Here's the drawing with two shaded views (mm, measured from the low corner). I have some questions. Coordinates: 2 decimals unless noted, no trailing zeros. Loops run counter-clockwise (first coordinate to the right, second up) from the corner with the lowest first, then second, coordinate; pieces in that order, holes last.
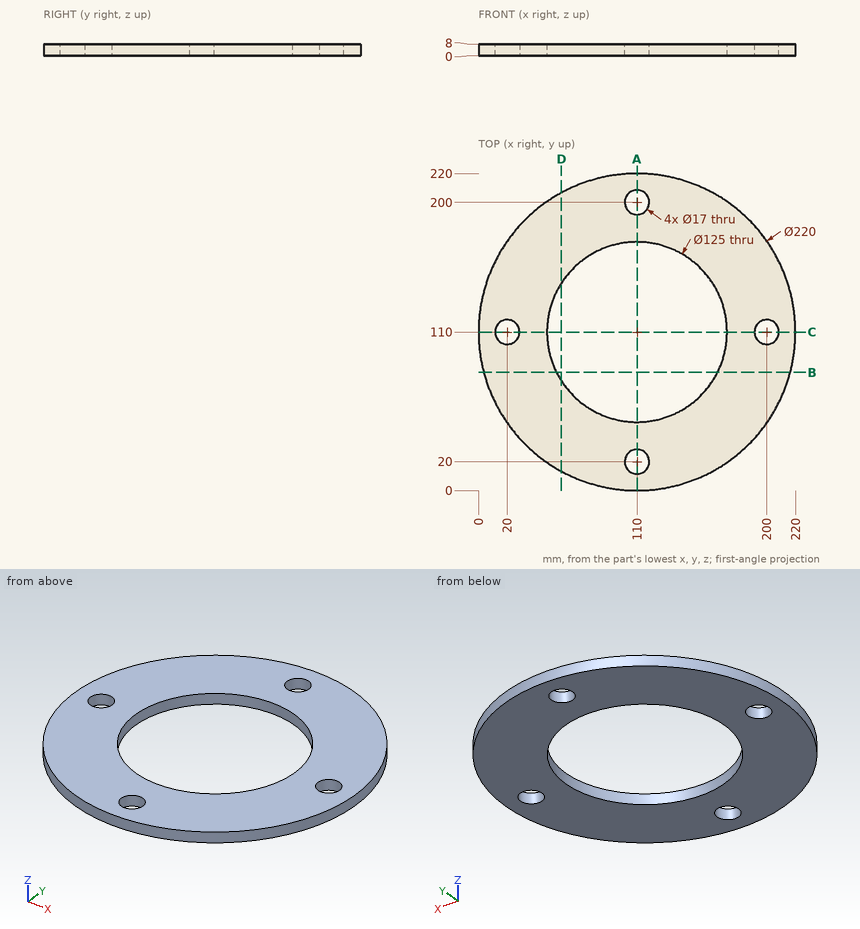
Q1. Will these pins go through, and if not, where does the flat tip stop? P1, Ø3, axis at y = 196.5, z = 6, coming from the -X side; P2, Ø13.5, axis at x = 110, y = 20, coming from the -Z side; P3, Ø1, axis at y = 34.5, z = 3.5, coming from the +X side; P4, Ø1.5, axis at x = 193.5, z = 6, coming from the +Y side.
Q2. Suppose I cut it at B-B on y = 82. Write out the boundary of the cut face in (x, z).
Q3. Suppose I cut it at A-A on x = 110. Write out the boundary of the cut face in (y, z), and give its area (3 significant figures).
Q4. Suppose I cut it at D-D on x = 57.5. Write out the boundary of the cut face in (y, z), and give its area (3 significant figures).
Q5. Please list where these lines run through material, in increasing order: probe 1 along X at (y, z) = (105, 6.75); probe 2 along X at (y, z) = (52, 1); probe 3 along X at (y, z) = (207, 6).
Check values:
1. P1: stops at x = 40.18
1. P2: passes through
1. P3: stops at x = 190.47
1. P4: stops at y = 182.47
2. outline: (3.62, 0) - (54.12, 0) - (54.12, 8) - (3.62, 8) - close; (165.88, 0) - (216.38, 0) - (216.38, 8) - (165.88, 8) - close
3. outline: (0, 0) - (11.5, 0) - (11.5, 8) - (0, 8) - close; (28.5, 0) - (47.5, 0) - (47.5, 8) - (28.5, 8) - close; (172.5, 0) - (191.5, 0) - (191.5, 8) - (172.5, 8) - close; (208.5, 0) - (220, 0) - (220, 8) - (208.5, 8) - close
3. area: 488 mm2
4. outline: (13.34, 0) - (76.09, 0) - (76.09, 8) - (13.34, 8) - close; (143.91, 0) - (206.66, 0) - (206.66, 8) - (143.91, 8) - close
4. area: 1,000 mm2
5. probe 1: x = 0.11 to 13.13, 26.87 to 47.7, 172.3 to 193.13, 206.87 to 219.89
5. probe 2: x = 16.53 to 86.71, 133.29 to 203.47
5. probe 3: x = 58.13 to 105.18, 114.82 to 161.87
